```python
from build123d import *

# Parameters (mm, degrees)
F0_R     = 3.175
F1_DEPTH = 3.048


with BuildPart() as f1:
    # F0 (on Front) → F1 (new body)
    with BuildSketch(Plane.XZ):
        with BuildLine():
            ThreePointArc((9.5102028503, 114.8307245366), (9.5213000643, 114.5654653895), (9.5250000939, 114.3))
            ThreePointArc((9.5250000939, 114.3), (-0.0114906805, 104.7750068372), (-9.5249723698, 114.3229813443))
            Line((-9.5249723698, 114.3229813443), (-15.747574407, 65.5073677534))
            ThreePointArc((-15.747574407, 65.5073677534), (0.0079100828, 79.3749980293), (15.7495670212, 65.4916735785))
            Line((15.7495670212, 65.4916735785), (9.5102028503, 114.8307245366))
        make_face()
        with Locations((-5.025569471, 99.6008760627)):
            Circle(F0_R, mode=Mode.SUBTRACT)
        with BuildLine():
            ThreePointArc((15.875, 63.5), (15.8436107227, 64.4978097358), (15.7495670212, 65.4916735785))
            ThreePointArc((15.7495670212, 65.4916735785), (0.0079100828, 79.3749980293), (-15.747574407, 65.5073677534))
            ThreePointArc((-15.747574407, 65.5073677534), (-15.8699038317, 63.9022155787), (-15.8290429523, 62.292927419))
            Line((-15.8290429523, 62.292927419), (-15.7035347362, 61.1730660111))
            ThreePointArc((-15.7035347362, 61.1730660111), (-0.5546795069, 47.6346933328), (15.5026829919, 60.0820408059))
            Line((15.5026829919, 60.0820408059), (15.875, 63.5))
        make_face()
        with Locations((0, 63.5)):
            Circle(F0_R, mode=Mode.SUBTRACT)
        with BuildLine():
            Line((9.9569104682, 9.1705224667), (15.5026829919, 60.0820408059))
            ThreePointArc((15.5026829919, 60.0820408059), (-0.5546795069, 47.6346933328), (-15.7035347362, 61.1730660111))
            Line((-15.7035347362, 61.1730660111), (-9.1457913245, 2.6608506249))
            ThreePointArc((-9.1457913245, 2.6608506249), (-5.7175616655, 7.6180780779), (0, 9.525))
            ThreePointArc((0, 9.525), (0.3388863295, 9.5189695375), (0.6773435479, 9.500885786))
            Line((0.6773435479, 9.500885786), (9.9569104682, 9.1705224667))
        make_face()
        with BuildLine():
            ThreePointArc((0, 9.525), (-5.7175616655, 7.6180780779), (-9.1457913245, 2.6608506249))
            ThreePointArc((-9.1457913245, 2.6608506249), (-7.6180780779, -5.7175616655), (0, -9.525))
            Line((0, -9.525), (0.6773435479, -9.500885786))
            ThreePointArc((0.6773435479, -9.500885786), (6.9705567315, -6.4912990883), (9.525, 0))
            ThreePointArc((9.525, 0), (9.4481631595, 1.207409587), (9.2188923022, 2.395339166))
            ThreePointArc((9.2188923022, 2.395339166), (6.0914751245, 7.3225375252), (0.6773435479, 9.500885786))
            Line((0.6773435479, 9.500885786), (0, 9.525))
        make_face()
        Circle(F0_R, mode=Mode.SUBTRACT)
        with BuildLine():
            Line((44.7324052746, 7.9324746146), (9.9569104682, 9.1705224667))
            Line((9.9569104682, 9.1705224667), (9.2188923022, 2.395339166))
            ThreePointArc((9.2188923022, 2.395339166), (9.4481631595, 1.207409587), (9.525, 0))
            ThreePointArc((9.525, 0), (6.9705567315, -6.4912990883), (0.6773435479, -9.500885786))
            Line((0.6773435479, -9.500885786), (44.7324052746, -7.9324746146))
            ThreePointArc((44.7324052746, -7.9324746146), (36.5125, 0), (44.7324052746, 7.9324746146))
        make_face()
        with BuildLine():
            Line((9.2188923022, 2.395339166), (9.9569104682, 9.1705224667))
            Line((9.9569104682, 9.1705224667), (0.6773435479, 9.500885786))
            ThreePointArc((0.6773435479, 9.500885786), (6.0914751245, 7.3225375252), (9.2188923022, 2.395339166))
        make_face()
        with BuildLine():
            ThreePointArc((52.3875, 0), (50.1616327839, 5.5119104847), (44.7324052746, 7.9324746146))
            ThreePointArc((44.7324052746, 7.9324746146), (36.5125, 0), (44.7324052746, -7.9324746146))
            ThreePointArc((44.7324052746, -7.9324746146), (50.1616327839, -5.5119104847), (52.3875, 0))
        make_face()
        with Locations((44.45, 0)):
            Circle(F0_R, mode=Mode.SUBTRACT)
        with BuildLine():
            ThreePointArc((-9.5249723698, 114.3229813443), (-0.0114906805, 104.7750068372), (9.5250000939, 114.3))
            ThreePointArc((9.5250000939, 114.3), (9.5213000643, 114.5654653895), (9.5102028503, 114.8307245366))
            ThreePointArc((9.5102028503, 114.8307245366), (-0.2539789795, 123.8216133857), (-9.5249723698, 114.3229813443))
        make_face()
        with Locations((0, 114.3)):
            Circle(F0_R, mode=Mode.SUBTRACT)
    extrude(amount=F1_DEPTH)


solid = f1.part
```
Input: part model. Units: mm. Frame: model coordinates. Give positions to 0.01 mm unless a question says otherwise; leave off trailing zeros. Write each loop counter-clockwise with the first axis right and the second up, starting at its lowest first coordinate (ties: lowest second). Pieces come first, ordered by that corner, then holes. Notation, with made-up numbers: (73, -26) - (132, -26) arc R20 cw to (132, -2) - close; hole circle Ø5 at (32, -4). An arc over 180 degrees is marked (long way). Write item = value, one per line. Start each with the question number.
1) Cut plane C-C (z = 59). Return loops of the section in (x, y).
2) Pin query (flat end, axial travel): pin 1 (5.5 mm diameter, centred on x = 0, z = 114.3, fed in from -Y); pin 2 (1.5 mm diameter, centred on y = -2, z = 14, fed in from -X); pin 3 (1.5 mm diameter, centred on y = -2, z = 105.5, fed in from -X). Return the tip coordinate at first contact, or that it passes through.
3) Draft query along Z for faces 1 (the face through (-0.048, -1.503, 123.825)), 2 (the face through (3, 0, 43)), 3 (the face through (12.875, -1.503, 35.955)). Return one class per face: pulls with the +Z half, pulls with the -Z half, needs draft (parallel to the pull), parting line crosses it, or undercut.
4) Cut plane A-A (y = -1.45). Give the number of separate pieces and of enclosed holes in the cut face, and give its area (3 significant figures).
5) Material intervals for L1, parallel to Z at x = 2, y = -2.2; L2, parallel to Z at x = 44.45, y = -0.75 (3 decimals); L3, parallel to X at y = -1.3, z = 88.5, sorted ascending. Write a range as [from, to].
6) Cut plane B-B (x = 26). Return loops of the section in (y, z), and give its area (3 significant figures).
Answers follow:
q1.outline = (-15.46, -3.05) - (15.38, -3.05) - (15.38, 0) - (-15.46, 0) - close
q2.pin_1 = through
q2.pin_2 = -10.5
q2.pin_3 = -10.75
q3.face_1 = pulls with the +Z half
q3.face_2 = needs draft
q3.face_3 = undercut
q4.separate_pieces = 1
q4.enclosed_holes = 6
q4.area = 3,720 mm^2
q5.L1 = [-9.45, -2.47], [2.47, 61.03], [65.97, 111.83], [116.77, 123.61]
q5.L2 = [-7.943, -3.175], [3.175, 7.943]
q5.L3 = [-12.82, 12.84]
q6.outline = (-3.05, -8.6) - (0, -8.6) - (0, 8.6) - (-3.05, 8.6) - close
q6.area = 52.4 mm^2
